Read the model definition and answer for the solid it produces. Units are mm, in the model's axes. Face numbers are marked on the shaded views. A direction names the side the tool comes from. Coordinates: 2 decimals unless noted, no trailing zeros. Loops run counter-clockwise (first coordinate to the right, second up) from the corner with the lowest first, then second, coordinate; pieces in that order, holes last. Notation, with made-up numbers: (-39, 71.5) -> (-26, 71.5) arc R23 cw to (-26, 79.5) -> close; hole circle Ø11 at (-16.75, 4). An arc over 180 degrees is marked (long way). Answer in a Markdown table with one row per item.
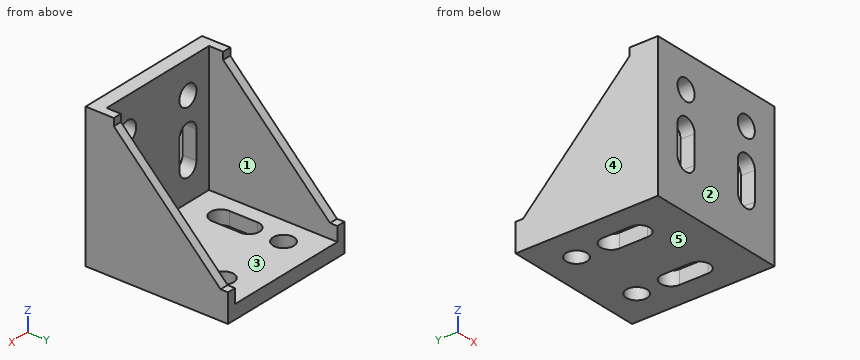
```python
from build123d import *

# Parameters (mm, degrees)
SKETCH_1_W               = 58
SKETCH_1_H               = 58
EXTRUDE_1_DEPTH          = 5.7
SKETCH_2_W               = 58
SKETCH_2_H               = 5.7
EXTRUDE_2_DEPTH          = 58
EXTRUDE_3_DEPTH          = 3.5
SKETCH_4_R               = 4.25
CUT_EXTRUDE_1_DEPTH      = 67.462696304
MIRROR_2_COPY_1_DEPTH    = 3.5
MIRROR_2_COPY_2_SKETCH_R = 4.25
MIRROR_2_COPY_2_DEPTH    = 67.462696304
MIRROR_2_COPY_3_DEPTH    = 3.5


with BuildPart() as part:
    # 草图1 → 凸台-拉伸1 (new body)
    with BuildSketch(Plane.XY):
        Rectangle(SKETCH_1_W, SKETCH_1_H)
    extrude(amount=EXTRUDE_1_DEPTH)

    # 草图2 → 凸台-拉伸2 (add)
    with BuildSketch(Plane(origin=(0, 0, 0), x_dir=(-1, 0, 0), z_dir=(0, 0, -1))):
        with Locations((0, -26.15)):
            Rectangle(SKETCH_2_W, SKETCH_2_H)
    extrude(amount=-EXTRUDE_2_DEPTH)

    # 草图3 → 凸台-拉伸3 (add)
    with BuildSketch(Plane.ZY.offset(29)):
        Polygon((5.7, 29), (11.5, 29), (11.5, 26), (55, -17.5), (58, -17.5), (58, -23.3), (5.7, -23.3), align=None)
    extrude_3 = extrude(amount=-EXTRUDE_3_DEPTH)

    # 草图4 → 切除-拉伸1 (cut, through all)
    with BuildSketch(Plane.XY.offset(5.7)):
        with Locations((-15, 15.651970491)):
            Circle(SKETCH_4_R)
        with BuildLine():
            Line((-19.25, -9.900882272), (-19.25, 1.599117728))
            ThreePointArc((-19.25, 1.599117728), (-15, 5.849117728), (-10.75, 1.599117728))
            Line((-10.75, 1.599117728), (-10.75, -9.900882272))
            ThreePointArc((-10.75, -9.900882272), (-15, -14.150882272), (-19.25, -9.900882272))
        make_face()
    cut_extrude_1 = extrude(amount=-CUT_EXTRUDE_1_DEPTH, mode=Mode.SUBTRACT)

    # 镜向1: 凸台-拉伸3, 切除-拉伸1 across plane
    add(extrude_3.mirror(Plane(origin=(0, 0, 0), x_dir=(0, 0, 1), z_dir=(1, 0, 0))))
    add(cut_extrude_1.mirror(Plane(origin=(0, 0, 0), x_dir=(0, 0, 1), z_dir=(1, 0, 0))), mode=Mode.SUBTRACT)

    # 镜向2: 切除-拉伸1 across plane
    add(cut_extrude_1.mirror(Plane(origin=(0, -14.5, 14.5), x_dir=(0, 0.7071067811865478, 0.7071067811865472), z_dir=(0, -0.7071067811865475, 0.7071067811865477))), mode=Mode.SUBTRACT)

    # 镜向2 copy 1 sketch → 镜向2 copy 1 (add)
    with BuildSketch(Plane(origin=(29, -29, 29), x_dir=(0, 1, 0), z_dir=(1, 0, 0))):
        Polygon((5.7, 29), (11.5, 29), (11.5, 26), (55, -17.5), (58, -17.5), (58, -23.3), (5.7, -23.3), align=None)
    extrude(amount=-MIRROR_2_COPY_1_DEPTH)

    # 镜向2 copy 2 sketch → 镜向2 copy 2 (cut, through all)
    with BuildSketch(Plane(origin=(0, -23.3, 29), x_dir=(-1, 0, 0), z_dir=(0, 1, 0))):
        with Locations((-15, 15.651970491)):
            Circle(MIRROR_2_COPY_2_SKETCH_R)
        with BuildLine():
            Line((-19.25, -9.900882272), (-19.25, 1.599117728))
            ThreePointArc((-19.25, 1.599117728), (-15, 5.849117728), (-10.75, 1.599117728))
            Line((-10.75, 1.599117728), (-10.75, -9.900882272))
            ThreePointArc((-10.75, -9.900882272), (-15, -14.150882272), (-19.25, -9.900882272))
        make_face()
    extrude(amount=-MIRROR_2_COPY_2_DEPTH, mode=Mode.SUBTRACT)

    # 镜向2 copy 3 sketch → 镜向2 copy 3 (add)
    with BuildSketch(Plane(origin=(-29, -29, 29), x_dir=(0, 1, 0), z_dir=(-1, 0, 0))):
        Polygon((5.7, -29), (11.5, -29), (11.5, -26), (55, 17.5), (58, 17.5), (58, 23.3), (5.7, 23.3), align=None)
    extrude(amount=-MIRROR_2_COPY_3_DEPTH)


solid = part.part
```
1. A cutting plane is placed at A-A on y = -5. Give the vertices of the cut face in (x, z), and give its area (3 significant figures).
A:
| item | result |
|---|---|
| outline | (-29, 0) -> (-19.25, 0) -> (-19.25, 5.7) -> (-25.5, 5.7) -> (-25.5, 42.5) -> (-29, 42.5) -> close; (-10.75, 0) -> (10.75, 0) -> (10.75, 5.7) -> (-10.75, 5.7) -> close; (19.25, 0) -> (29, 0) -> (29, 42.5) -> (25.5, 42.5) -> (25.5, 5.7) -> (19.25, 5.7) -> close |
| area | 491 mm2 |
2. The mould has two halves that part along X. Classify the marked faces 3, 4 and 5: pulls with the +X half, pulls with the -X half, needs draft (parallel to the pull), parting line crosses it, or undercut.
A:
| item | result |
|---|---|
| face 3 | undercut |
| face 4 | pulls with the -X half |
| face 5 | needs draft |
3. Given pin 1 Ø0.9 at (x, y) = (28, 27) entering from +Z; pin 2 Ø2 at (x, y) = (-15.5, -12.5) entering from +Z; pin 3 Ø1 at (x, y) = (-22, -3) entering from +Z; pin 4 Ø13.5 at (x, y) = (15, 15.65) entering from -Z, each flat-ended and moving along its own axis, determine where each tip first touches the part or whether it passes through.
A:
| item | result |
|---|---|
| pin 1 | stops at z = 11.5 |
| pin 2 | passes through |
| pin 3 | stops at z = 5.7 |
| pin 4 | stops at z = 0 |
4. A cutting plane is placed at D-D on y = 8. Give the vertices of the cut face in (x, z), and give its area (3 significant figures).
A:
| item | result |
|---|---|
| outline | (-29, 0) -> (29, 0) -> (29, 29.5) -> (25.5, 29.5) -> (25.5, 5.7) -> (-25.5, 5.7) -> (-25.5, 29.5) -> (-29, 29.5) -> close |
| area | 497 mm2 |
5. Find the intervals of material crossed by probe 1 along X at (y, z) = (3, 32); probe 2 along Y at (x, z) = (-15, 2.15); probe 3 along Z at (x, y) = (-15, -26), in increasing order.
A:
| item | result |
|---|---|
| probe 1 | x = -29 to -25.5, 25.5 to 29 |
| probe 2 | y = -29 to -14.15, 5.85 to 11.4, 19.9 to 29 |
| probe 3 | z = 0 to 14.85, 34.85 to 40.4, 48.9 to 58 |
6. A cutting plane is placed at C-C on x = 15. Give the vertices of the cut face in (y, z), and give its area (3 significant figures).
A:
| item | result |
|---|---|
| outline | (-29, 0) -> (-14.15, 0) -> (-14.15, 5.7) -> (-23.3, 5.7) -> (-23.3, 14.85) -> (-29, 14.85) -> close; (-29, 34.85) -> (-23.3, 34.85) -> (-23.3, 40.4) -> (-29, 40.4) -> close; (-29, 48.9) -> (-23.3, 48.9) -> (-23.3, 58) -> (-29, 58) -> close; (5.85, 0) -> (11.4, 0) -> (11.4, 5.7) -> (5.85, 5.7) -> close; (19.9, 0) -> (29, 0) -> (29, 5.7) -> (19.9, 5.7) -> close |
| area | 304 mm2 |
7. A cutting plane is placed at B-B on z = 27. Give the vertices of the cut face in (x, y).
A:
| item | result |
|---|---|
| outline | (-29, -29) -> (-19.25, -29) -> (-19.25, -23.3) -> (-25.5, -23.3) -> (-25.5, 10.5) -> (-29, 10.5) -> close; (-10.75, -29) -> (10.75, -29) -> (10.75, -23.3) -> (-10.75, -23.3) -> close; (19.25, -29) -> (29, -29) -> (29, 10.5) -> (25.5, 10.5) -> (25.5, -23.3) -> (19.25, -23.3) -> close |
8. A tool of negligible diameter and unlimited length cuts with its end or side. For the marked faces 1 and 2, from which of +Z, -Z, +X, -X, +Y, -Y can it reach the whole face along a straight path? Write none if from no direction.
A:
| item | result |
|---|---|
| face 1 | +Z, +Y |
| face 2 | +Z, -Z, +X, -X, -Y |
